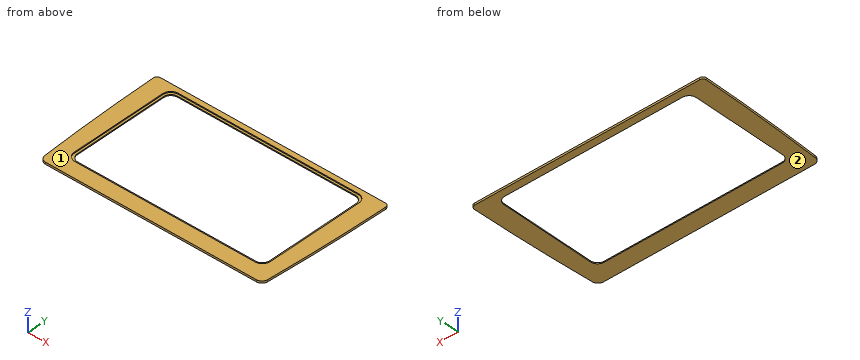
from build123d import *

# Parameters (mm, degrees)
PAD_DEPTH       = 2
FILLET_R        = 3.5
FILLET001_R     = 6
POCKET_DEPTH    = 1
POCKET001_DEPTH = 5


with BuildPart() as part:
    # Sketch → Pad (new body)
    with BuildSketch(Plane.XY):
        with BuildLine():
            Line((-114.5, 111), (114.5, 111))
            ThreePointArc((109.5, -20), (112.998546, 45.461888), (114.5, 111))
            Line((109.5, -20), (-109.5, -20))
            ThreePointArc((-114.5, 111), (-112.998546, 45.461888), (-109.5, -20))
        make_face()
    extrude(amount=PAD_DEPTH)

    # Fillet
    fillet_edges = [part.edges().sort_by_distance(p)[0] for p in [
        (114.5, 111, 1),
        (-114.5, 111, 1),
    ]]
    fillet(fillet_edges, radius=FILLET_R)

    # Fillet001
    fillet001_edges = [part.edges().sort_by_distance(p)[0] for p in [
        (109.5, -20, 1),
        (-109.5, -20, 1),
    ]]
    fillet(fillet001_edges, radius=FILLET001_R)

    # Sketch001 (on Face5 of Fillet001) → Pocket (cut)
    with BuildSketch(Plane.XY.offset(2)):
        with BuildLine():
            Line((-88.75, 106), (88.75, 106))
            ThreePointArc((96.75, 98), (94.406854, 103.656854), (88.75, 106))
            Line((96.75, 98), (96.75, 3))
            ThreePointArc((88.75, -5), (94.406854, -2.656854), (96.75, 3))
            Line((88.75, -5), (-88.75, -5))
            ThreePointArc((-96.75, 3), (-94.406854, -2.656854), (-88.75, -5))
            Line((-96.75, 3), (-96.75, 98))
            ThreePointArc((-88.75, 106), (-94.406854, 103.656854), (-96.75, 98))
        make_face()
    extrude(amount=-POCKET_DEPTH, mode=Mode.SUBTRACT)

    # Sketch002 (on Face19 of Pocket) → Pocket001 (cut)
    with BuildSketch(Plane.XY.offset(1)):
        with BuildLine():
            Line((-87.75, 104), (87.75, 104))
            ThreePointArc((94.75, 97), (92.699747, 101.949747), (87.75, 104))
            Line((94.75, 97), (94.75, 4))
            ThreePointArc((87.75, -3), (92.699747, -0.949747), (94.75, 4))
            Line((87.75, -3), (-87.75, -3))
            ThreePointArc((-94.75, 4), (-92.699747, -0.949747), (-87.75, -3))
            Line((-94.75, 4), (-94.75, 97))
            ThreePointArc((-87.75, 104), (-92.699747, 101.949747), (-94.75, 97))
        make_face()
    extrude(amount=-POCKET001_DEPTH, mode=Mode.SUBTRACT)


solid = part.part
For this review, take the finished solid that the model builds, in its own axes (mm). Face numbers are marked on the shaded views. Round coordinates to 2 decimals unless told otherwise and drop trailing zeros. Order: outer loops, then holes, each group sorted by start corner. A loop starts at its lowest first (then second) coordinate and runs counter-clockwise, first axis right, second up. Notation, with made-up numbers: (22.5, 25) -> (27.5, 25) arc R16 ccw to (27.5, 47) -> close; hole circle Ø2 at (16, -6.75). An arc over 180 degrees is marked (long way). Put each result on its own line as item: value.
Q1. Insertion check: pin 1 Ø0.5 at (y, z) = (74, 1.5) entering from -X. The pin has a flat end and moves straight along its axis. Give the tip position at first contact, or say it passes through.
Check result:
pin 1: x = -113.9
Q2. Mouldability with a two-part tool opening along Z and no side actions: class the marked faces 1 and 2 as pulls with the +Z half, pulls with the -Z half, needs draft (parallel to the pull), parting line crosses it, or undercut.
Check result:
face 1: pulls with the +Z half
face 2: pulls with the -Z half
Q3. For probe 1 along Y at (x, z) = (79, 0.4); probe 2 along Y at (x, z) = (-39, 1.6); probe 3 along Z at (x, y) = (49, -4), list the stretches that pass through material, from the lowest coordinate up. Write a range as [from, to].
Check result:
probe 1: [-20, -3], [104, 111]
probe 2: [-20, -5], [106, 111]
probe 3: [0, 1]
Q4. Add section C-C on z = 0.45. Write out the cut boundary in (x, y).
Check result:
outline: (-114.47, 107.47) arc R2150.31 ccw to (-109.88, -14.4) arc R6 ccw to (-103.89, -20) -> (103.89, -20) arc R6 ccw to (109.88, -14.4) arc R2150.31 ccw to (114.47, 107.47) arc R3.5 ccw to (110.97, 111) -> (-110.97, 111) arc R3.5 ccw to start; hole (-94.75, 4) arc R7 ccw to (-87.75, -3) -> (87.75, -3) arc R7 ccw to (94.75, 4) -> (94.75, 97) arc R7 ccw to (87.75, 104) -> (-87.75, 104) arc R7 ccw to (-94.75, 97) -> close
Q5. Add section A-A on x = 66.5. Write out the cut boundary in (y, z).
Check result:
outline: (-20, 0) -> (-3, 0) -> (-3, 1) -> (-5, 1) -> (-5, 2) -> (-20, 2) -> close; (104, 0) -> (111, 0) -> (111, 2) -> (106, 2) -> (106, 1) -> (104, 1) -> close
Q6. Add section B-B on y = 25.5. Write out the cut boundary in (x, z), plus the area to 3 significant figures.
Check result:
outline: (-112.14, 0) -> (-94.75, 0) -> (-94.75, 1) -> (-96.75, 1) -> (-96.75, 2) -> (-112.14, 2) -> close; (94.75, 0) -> (112.14, 0) -> (112.14, 2) -> (96.75, 2) -> (96.75, 1) -> (94.75, 1) -> close
area: 65.6 mm2
